Geometry check sheet. Reference: the model listing, model coordinates, mm. Face numbers are marked on the shaded views. A direction names the side the tool comes from. Round coordinates to 2 decimals unless told otherwise and drop trailing zeros. Write each loop counter-clockwise with the first axis right and the second up, starting at its lowest first coordinate (ties: lowest second). Pieces come first, ordered by that corner, then holes. Notation, with made-up numbers: M 68.5,-38.75 L 100.5,-38.75 A30 cw 100.5,-1.75 Z; hole C -20,3.5 d2. An arc over 180 degrees is marked long. Use a Markdown table: item, result.
```python
from build123d import *

# Parameters (mm, degrees)
F1_DEPTH = 94.3762343377
F3_DEPTH = 45.3802291304
F5_DEPTH = 38.9628577977


with BuildPart() as f1:
    # F0 (on Front) → F1 (new body)
    with BuildSketch(Plane.XZ):
        Polygon((-20.9776982665, 37.0258837938), (-44.0754815936, 37.0258837938), (-45.3320667148, -51.1417090893), (48.8735437393, -51.1417090893), (49.6917665005, 36.9159281254), (18.4360146523, 36.9159281254), (18.4360146523, -26.4765024185), (-22.8313431144, -24.2851227522), align=None)
    extrude(amount=F1_DEPTH)

    # F2 (on face) → F3 (join)
    with BuildSketch(Plane(origin=(-44.5941249017, 0, 0.635565881), x_dir=(0, -1, 0), z_dir=(-0.9998984524, 0, 0.0142507862))):
        Polygon((0, -51.7825333627), (94.3762343377, 36.394013638), (0, 36.394013638), align=None)
    extrude(amount=F3_DEPTH)

    # F4 (on face) → F5 (join)
    with BuildSketch(Plane(origin=(49.3444870134, 0, -0.45850404), x_dir=(0, 1, 0), z_dir=(0.9999568331, 0, -0.0092914989))):
        Polygon((0, -50.685392981), (-94.3762343377, 37.3760455736), (-94.3762343377, -50.685392981), align=None)
    extrude(amount=F5_DEPTH)


solid = f1.part
```
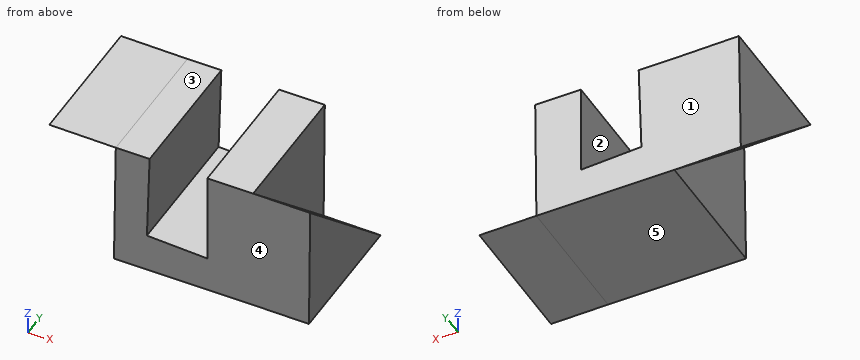
Item 1: Cross-section at C-C, the plane z = -34. Record the cut outline in (x, y), and give its area (3 significant figures).
Outcome:
| item | result |
|---|---|
| outline | M -90.47,-17.66 L -45.09,-18.35 L -45.09,-94.38 L 88,-94.38 L 88,-18.76 L 49.03,-18.37 L 49.03,0 L -90.47,0 Z |
| area | 12,700 mm2 |
Item 2: Cross-section at D-D, the plane z = 4. Record the cut outline in (x, y), and give its area (3 significant figures).
Outcome:
| item | result |
|---|---|
| outline | M -89.93,-58.33 L -44.55,-59.02 L -44.55,-94.38 L -21.98,-94.38 L -21.98,0 L -89.93,0 Z; M 18.44,-94.38 L 88.35,-94.38 L 88.35,-59.49 L 49.39,-59.1 L 49.39,0 L 18.44,0 Z |
| area | 9,080 mm2 |
Item 3: Material ranges on line 1 along Z through (x, y) = (-30, -65); line 2 along X through (y, z) = (-21, -12); line 3 along X through (y, z) = (-32.5, 27), recorded low to high. Write a range as from..to.
Outcome:
| item | result |
|---|---|
| line 1 | z = -51.14..37.03 |
| line 2 | x = -90.16..-22.46, 18.44..49.24 |
| line 3 | x = -89.6..-21.28, 18.44..49.6 |
Item 4: Cross-section at A-A, the plane z = -20. Record the cut outline in (x, y), and give its area (3 significant figures).
Outcome:
| item | result |
|---|---|
| outline | M -90.27,-32.64 L -44.89,-33.33 L -44.89,-94.38 L -22.7,-94.38 L -22.7,0 L -90.27,0 Z; M 18.44,-94.38 L 88.13,-94.38 L 88.13,-33.76 L 49.16,-33.38 L 49.16,0 L 18.44,0 Z |
| area | 8,860 mm2 |
Item 5: Go/stop test with flat-tipped pins: pin 1 (4 mm diameter, centred on x = 7, y = -32.5, fed in from -Z); pin 2 (7 mm diameter, centred on x = -31, y = -38.5, fed in from +Z); pin 3 (1 mm diameter, centred on y = -11.5, z = -20.5, fed in from +X). Record where each tip stops, or that it passes through.
Outcome:
| item | result |
|---|---|
| pin 1 | stops at z = -51.14 |
| pin 2 | stops at z = 37.03 |
| pin 3 | stops at x = 49.16 |
Item 6: Access from +Z, -Z, +X, -X, +Y, -Y to the whole of each face (thin tool, end or side, straight path). Record for the marked faces 1, 2, 3, 4 and 5.
Outcome:
| item | result |
|---|---|
| face 1 | +Z, -Z, +X, -X, +Y |
| face 2 | +Z, +Y, -Y |
| face 3 | +Z, +X, +Y, -Y |
| face 4 | +Z, -Z, +X, -X, -Y |
| face 5 | -Z, -X, +Y, -Y |
Item 7: Cross-section at B-B, the plane y = -22. Record the cut outline in (x, z), and give its area (3 significant figures).
Outcome:
| item | result |
|---|---|
| outline | M -90.41,-29.94 L -45.04,-30.59 L -45.33,-51.14 L 48.87,-51.14 L 87.83,-51.5 L 88.03,-30.98 L 49.06,-30.61 L 49.69,36.92 L 18.44,36.92 L 18.44,-26.48 L -22.83,-24.29 L -20.98,37.03 L -44.08,37.03 L -89.45,37.67 Z |
| area | 9,630 mm2 |
